The model under review builds one solid part; all positions refer to its coordinate system, in mm. A direction names the side the tool comes from. Round coordinates to 2 decimals unless told otherwise and drop trailing zeros. Order: outer loops, then holes, each group sorted by start corner. A loop starts at its lowest first (then second) coordinate and runs counter-clockwise, first axis right, second up. Notation, with made-up numbers: (17.5, -13.75) -> (71.5, -13.75) arc R32 cw to (71.5, 25.25) -> close; hole circle Ø10 at (77, 26.5). An arc over 180 degrees is marked (long way). Use a Markdown table: item, result. Add a question column.
```python
from build123d import *

# Parameters (mm, degrees)
CROQUIS1_W              = 150
CROQUIS1_H              = 80
SALIENTE_EXTRUIR1_DEPTH = 6
CROQUIS2_R              = 6.5
CORTAR_EXTRUIR1_DEPTH   = 6
CROQUIS3_W              = 6
CROQUIS3_H              = 16
CORTAR_EXTRUIR2_DEPTH   = 6


with BuildPart() as part:
    # Croquis1 → Saliente-Extruir1 (new body)
    with BuildSketch(Plane(origin=(0, 0, 0), x_dir=(0, 0, -1), z_dir=(1, 0, 0))):
        Rectangle(CROQUIS1_W, CROQUIS1_H)
    extrude(amount=SALIENTE_EXTRUIR1_DEPTH)

    # Croquis2 → Cortar-Extruir1 (cut)
    with BuildSketch(Plane(origin=(6, 0, 0), x_dir=(0, 0, -1), z_dir=(1, 0, 0))):
        with Locations((-43.61, 0)):
            Circle(CROQUIS2_R)
        with Locations((5, 0)):
            Circle(CROQUIS2_R)
        with Locations((43.1, 0)):
            Circle(CROQUIS2_R)
    extrude(amount=-CORTAR_EXTRUIR1_DEPTH, mode=Mode.SUBTRACT)

    # Croquis3 → Cortar-Extruir2 (cut)
    with BuildSketch(Plane(origin=(6, 0, 0), x_dir=(0, 0, -1), z_dir=(1, 0, 0))):
        with Locations((-72, 32)):
            Rectangle(CROQUIS3_W, CROQUIS3_H)
        with Locations((-72, -32)):
            Rectangle(CROQUIS3_W, CROQUIS3_H)
        with Locations((72, -32)):
            Rectangle(CROQUIS3_W, CROQUIS3_H)
        with Locations((72, 32)):
            Rectangle(CROQUIS3_W, CROQUIS3_H)
        with Locations((72, 0)):
            Rectangle(CROQUIS3_W, CROQUIS3_H)
        with Locations((-72, 0)):
            Rectangle(CROQUIS3_W, CROQUIS3_H)
    extrude(amount=-CORTAR_EXTRUIR2_DEPTH, mode=Mode.SUBTRACT)


solid = part.part
```
Q1. Wall thickness on line 1 (Y direction, x = 3.9, z = -5); line 2 (Z direction, x = 4.1, y = -1); line 3 (Y direction, x = 4.2, z = -2.5): over which ranges is each line inside the solid? List them lowest first. Write a range as [from, to].
Q2. Add section D-D (y = -26). Write out the cut boundary in (x, z).
Q3. Add section B-B (y = 0). Write out the cut boundary in (x, z), then the cut area to 3 significant figures.
Q4. Machinability: for faces 1 (the flat face through (3, 32, -69)), 2 (the flat face through (3, -8, 72)), 3 (the flat face through (3, -8, -72)), which of the approach directions +Z, -Z, +X, -X, +Y, -Y give a long, thin tool a straight path to every point of the face, cutting with its end or side? Answer none if there is none.
Q5. Add section C-C (x = 3.9). Write out the cut boundary in (y, z).
Q6. Mouldability with a two-part tool opening along Y and no side actions: class faces 4 (the flat face through (3, -16, -75)), 5 (the cylindrical face through (3.042, 0.286, 50.104)), 6 (the flat face through (3, 24, 72)) as pulls with the +Y half, pulls with the -Y half, needs draft (parallel to the pull), parting line crosses it, or undercut.
Q7. Insertion check: pin 1 (1.8 mm diameter, centred on x = 2, z = 72, fed in from +Y); pin 2 (3 mm diameter, centred on x = 3.5, y = 33, fed in from +Z); pin 3 (1.8 mm diameter, centred on x = 2, z = 73.5, fed in from -Y). Each pin has a flat end and moves straight along its axis. Give the tip position at first contact, or say it passes through.
Q8. Add section A-A (z = -43.1). Write out the cut boundary in (x, y).
Report:
| question | item | result |
|---|---|---|
| 1 | line 1 | y = [-40, -6.5], [6.5, 40] |
| 1 | line 2 | z = [-69, -49.52], [-36.68, -11.42], [1.42, 37.19], [50.03, 69] |
| 1 | line 3 | y = [-40, -6], [6, 40] |
| 2 | outline | (0, -69) -> (6, -69) -> (6, 69) -> (0, 69) -> close |
| 3 | outline | (0, -69) -> (6, -69) -> (6, -49.6) -> (0, -49.6) -> close; (0, -36.6) -> (6, -36.6) -> (6, -11.5) -> (0, -11.5) -> close; (0, 1.5) -> (6, 1.5) -> (6, 37.11) -> (0, 37.11) -> close; (0, 50.11) -> (6, 50.11) -> (6, 69) -> (0, 69) -> close |
| 3 | area | 594 mm² |
| 4 | face 1 | -Z, +X, -X, +Y |
| 4 | face 2 | +Z, +X, -X |
| 4 | face 3 | -Z, +X, -X |
| 5 | outline | (-40, -69) -> (-24, -69) -> (-24, -75) -> (-8, -75) -> (-8, -69) -> (8, -69) -> (8, -75) -> (24, -75) -> (24, -69) -> (40, -69) -> (40, 69) -> (24, 69) -> (24, 75) -> (8, 75) -> (8, 69) -> (-8, 69) -> (-8, 75) -> (-24, 75) -> (-24, 69) -> (-40, 69) -> close; hole circle Ø13 at (0, -43.1); hole circle Ø13 at (0, -5); hole circle Ø13 at (0, 43.61) |
| 6 | face 4 | needs draft |
| 6 | face 5 | undercut |
| 6 | face 6 | pulls with the +Y half |
| 7 | pin 1 | stops at y = 24 |
| 7 | pin 2 | stops at z = 69 |
| 7 | pin 3 | stops at y = -24 |
| 8 | outline | (0, -40) -> (6, -40) -> (6, -6.5) -> (0, -6.5) -> close; (0, 6.5) -> (6, 6.5) -> (6, 40) -> (0, 40) -> close |
